The drawing under review shows one solid part. Ordinate dimensions are in mm from its lowest x, y, z. Round coordinates to 2 decimals unless told otherwise and drop trailing zeros. Order: outer loops, then holes, each group sorted by start corner. A loop starts at its lowest first (then second) coordinate and runs counter-clockwise, first axis right, second up. Notation, with made-up numbers: (-39.75, -10) -> (19.25, -10) arc R28 cw to (19.25, 14) -> close; hole circle Ø10 at (56, 34). An arc over 180 degrees is marked (long way). Return JSON: item names as keys, results as strings. Group by question number.
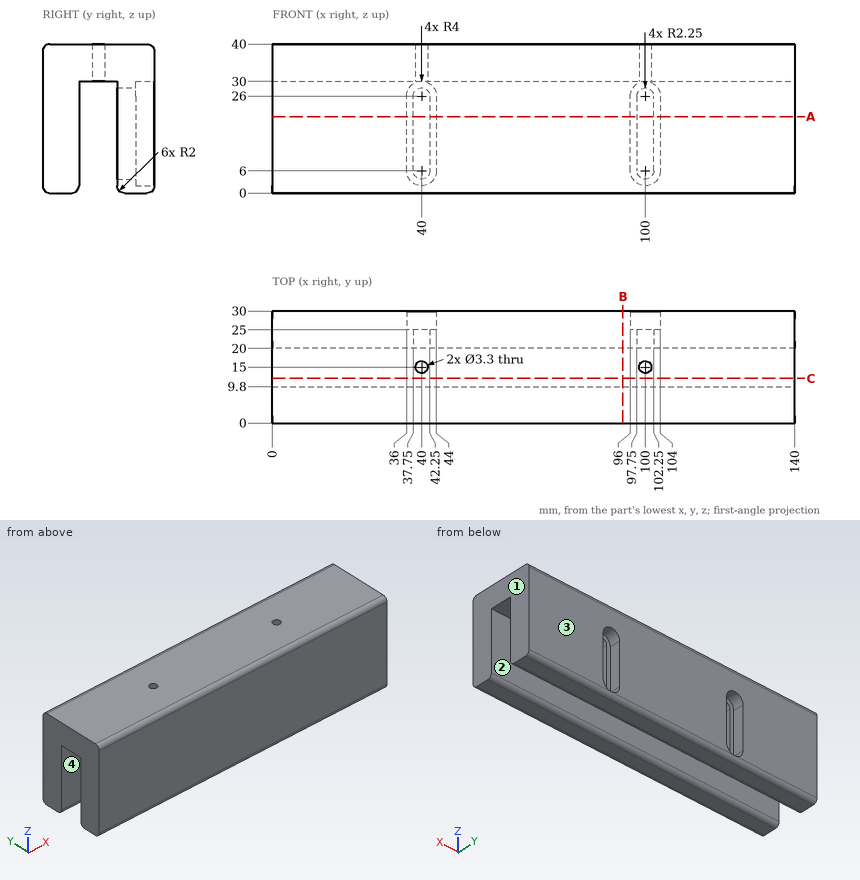
Item 1: Consider section B-B on x = 94. State the section outline as (y, z) points, plus the area to 3 significant figures.
Item 2: Consider section C-C on y = 12. State the section outline as (x, z) points, plus the area to 3 significant figures.
Item 3: Wall thickness on line 1 along X through (y, z) = (25.25, 20); line 2 along Y through (x, z) = (100, 35.5); line 3 along Y through (x, z) = (81.5, 15.5): over which ranges is each line inside the solid? List them lowest first.
Item 4: Insertion check: pin 1 Ø2 at (x, y) = (40, 15) entering from +Z; pin 2 Ø1 at (x, y) = (92.5, 15) entering from -Z. Each pin has a flat end and moves straight along its axis. Give the tip position at first contact, or say it passes through.
Item 5: The part is to be moulded in two halves that separate along Y. For the marked faces 1, 2, 3 and 4, say which applies: +Y half, -Y half, draft (parallel to the pull), parting line (faces both ways), or undercut.
Item 6: Consider section A-A on z = 20.5. State the section outline as (x, y) points, plus the area to 3 significant figures.
Values:
{
 "1": {"outline": "(0, 2) arc R2 ccw to (2, 0) -> (7.8, 0) arc R2 ccw to (9.8, 2) -> (9.8, 30) -> (20, 30) -> (20, 2) arc R2 ccw to (22, 0) -> (28, 0) arc R2 ccw to (30, 2) -> (30, 38) arc R2 ccw to (28, 40) -> (2, 40) arc R2 ccw to (0, 38) -> close", "area": "889 mm^2"},
 "2": {"outline": "(0, 30) -> (140, 30) -> (140, 40) -> (0, 40) -> close", "area": "1,400 mm^2"},
 "3": {"line 1": "0 to 36, 44 to 96, 104 to 140", "line 2": "0 to 13.35, 16.65 to 30", "line 3": "0 to 9.8, 20 to 30"},
 "4": {"pin 1": "through", "pin 2": "z = 30"},
 "5": {"face 1": "draft", "face 2": "undercut", "face 3": "+Y half", "face 4": "undercut"},
 "6": {"outline": "(0, 0) -> (140, 0) -> (140, 9.8) -> (0, 9.8) -> close; (0, 20) -> (37.75, 20) -> (37.75, 25) -> (36, 25) -> (36, 30) -> (0, 30) -> close; (42.25, 20) -> (97.75, 20) -> (97.75, 25) -> (96, 25) -> (96, 30) -> (44, 30) -> (44, 25) -> (42.25, 25) -> close; (102.25, 20) -> (140, 20) -> (140, 30) -> (104, 30) -> (104, 25) -> (102.25, 25) -> close", "area": "2,650 mm^2"}
}
